Here's the drawing with two shaded views (mm, measured from the low corner). I have some questions. Round coordinates to 2 decimals unless told otherwise and drop trailing zeros. Write each loop counter-clockwise with the first axis right and the second up, starting at its lowest first coordinate (ties: lowest second). Pieces come first, ordered by that corner, then holes. Notation, with made-up numbers: (52, 21) -> (71, 21) arc R26 ccw to (71, 60) -> close; hole circle Ø4 at (0, -21). An arc over 180 degrees is marked (long way). Use CSV: the item, a comma, the result in double quotes.
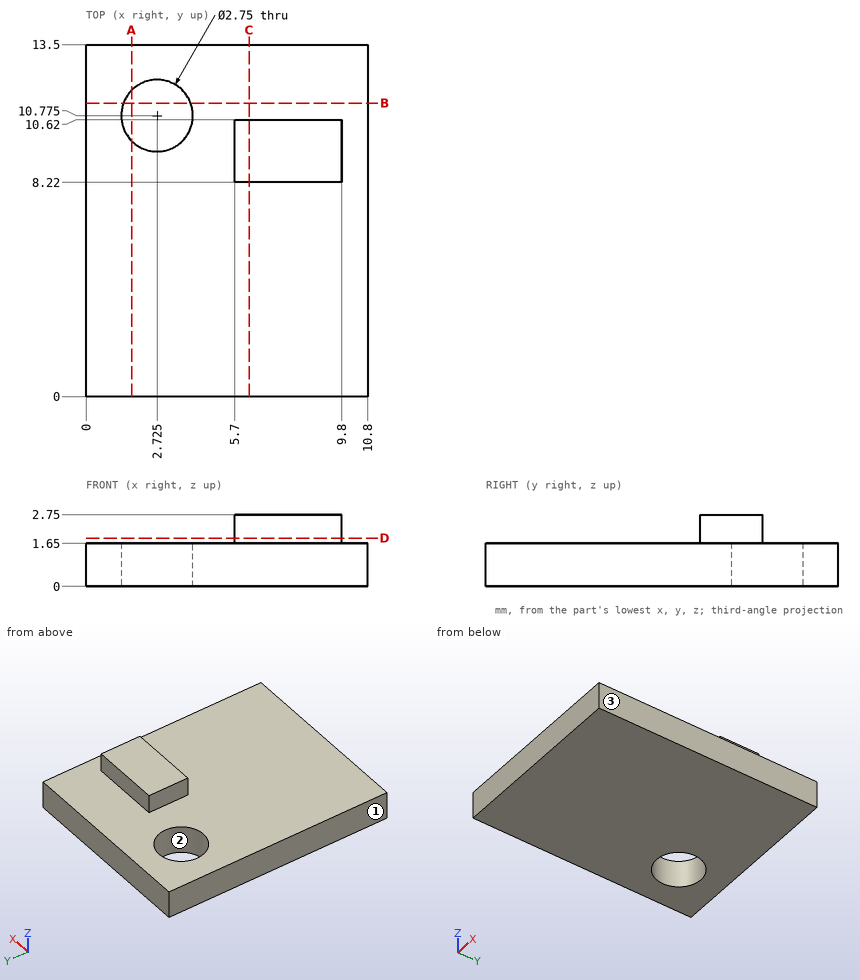
Q1. Suppose I cut it at B-B (y = 11.25). Write out the boundary of the cut face in (x, z), and give its area (3 significant figures).
Resolved:
outline,"(0, 0) -> (1.43, 0) -> (1.43, 1.65) -> (0, 1.65) -> close; (4.02, 0) -> (10.8, 0) -> (10.8, 1.65) -> (4.02, 1.65) -> close"
area,"13.6 mm^2"
Q2. Suppose I cut it at A-A (x = 1.75). Write out the boundary of the cut face in (y, z), and give its area (3 significant figures).
Resolved:
outline,"(0, 0) -> (9.81, 0) -> (9.81, 1.65) -> (0, 1.65) -> close; (11.74, 0) -> (13.5, 0) -> (13.5, 1.65) -> (11.74, 1.65) -> close"
area,"19.1 mm^2"
Q3. Suppose I cut it at D-D (z = 1.85). Write out the boundary of the cut face in (x, y).
Resolved:
outline,"(5.7, 8.22) -> (9.8, 8.22) -> (9.8, 10.62) -> (5.7, 10.62) -> close"
Q4. If we mould it in two halves opening along X, with no side actions, what happens to the marked faces 1, 2 and 3? For each: released by +X, released by -X, zero draft, split by the parting line, or undercut.
Resolved:
face 1,"released by -X"
face 2,"undercut"
face 3,"released by +X"
Q5. Please list where these lines run through material, in increasing order: probe 1 along Z at (x, y) = (5.25, 6.75); probe 2 along Y at (x, z) = (1.75, 0.8); probe 3 along X at (y, z) = (12, 0.9).
Resolved:
probe 1,"z = 0 to 1.65"
probe 2,"y = 0 to 9.81, 11.74 to 13.5"
probe 3,"x = 0 to 2.1, 3.35 to 10.8"
Q6. Suppose I cut it at C-C (x = 6.25). Write out the boundary of the cut face in (y, z).
Resolved:
outline,"(0, 0) -> (13.5, 0) -> (13.5, 1.65) -> (10.62, 1.65) -> (10.62, 2.75) -> (8.22, 2.75) -> (8.22, 1.65) -> (0, 1.65) -> close"
Q7. Will these pins go through, and if not, where does the flat tip stop? P1, Ø3, axis at x = 9.5, y = 2.5, coming from the +Z side; P2, Ø4.5, axis at x = 2.725, y = 10.775, coming from the -Z side; P3, Ø0.6, axis at x = 8, z = 2.5, coming from the +Y side.
Resolved:
P1,"stops at z = 1.65"
P2,"stops at z = 0"
P3,"stops at y = 10.62"
